Read the model definition and answer for the solid it produces. Units are mm, in the model's axes. A direction names the side the tool comes from. Coordinates: 2 decimals unless noted, no trailing zeros. Write each loop counter-clockwise with the first axis right and the second up, starting at its lowest first coordinate (ties: lowest second). Pieces come first, ordered by that corner, then holes. Notation, with made-up numbers: M -7,-13.5 L 32,-13.5 A28 cw 32,21.5 Z; hole C -2.5,11 d7. An arc over 180 degrees is marked long. Use a Markdown table: item, result. Add a question column.
from build123d import *

# Parameters (mm, degrees)
F1_DEPTH = 1.905
F3_DEPTH = 0.762
F4_R     = 4.445
F5_DEPTH = 3.048
F6_W     = 15.5236069113
F6_H     = 4.7940094955
F7_DEPTH = 0.762
F8_R     = 1.905
F9_DEPTH = 1.524


with BuildPart() as f1:
    # F0 (on Top) → F1 (new body)
    with BuildSketch(Plane.XY):
        with BuildLine():
            ThreePointArc((0, 10.16), (1.7642654851, 10.0056467706), (3.4749246562, 9.5472770272))
            Line((3.4749246562, 9.5472770272), (4.3436558202, 11.934096284))
            ThreePointArc((4.3436558202, 11.934096284), (2.2053318564, 12.5070584633), (0, 12.7))
            Line((0, 12.7), (0, 10.16))
        make_face()
        with BuildLine():
            ThreePointArc((-3.4749246562, 9.5472770272), (-1.7642654851, 10.0056467706), (0, 10.16))
            Line((0, 10.16), (0, 12.7))
            ThreePointArc((0, 12.7), (-2.2053318564, 12.5070584633), (-4.3436558202, 11.934096284))
            Line((-4.3436558202, 11.934096284), (-3.4749246562, 9.5472770272))
        make_face()
        with BuildLine():
            Line((4.3436558202, -11.934096284), (3.4749246562, -9.5472770272))
            ThreePointArc((3.4749246562, -9.5472770272), (0, -10.16), (-3.4749246562, -9.5472770272))
            Line((-3.4749246562, -9.5472770272), (-4.3436558202, -11.934096284))
            ThreePointArc((-4.3436558202, -11.934096284), (0, -12.7), (4.3436558202, -11.934096284))
        make_face()
        with BuildLine():
            Line((0, 0), (-1.5202795371, 4.1769336994))
            ThreePointArc((-1.5202795371, 4.1769336994), (-3.6411308369, 2.5495472596), (-4.445, 0))
            Line((-4.445, 0), (0, 0))
        make_face()
        with BuildLine():
            ThreePointArc((1.5202795371, -4.1769336994), (3.6411308369, -2.5495472596), (4.445, 0))
            ThreePointArc((4.445, 0), (3.6411308369, 2.5495472596), (1.5202795371, 4.1769336994))
            ThreePointArc((1.5202795371, 4.1769336994), (0.7718661497, 4.3774704621), (0, 4.445))
            Line((0, 4.445), (0, 0))
            Line((0, 0), (-4.445, 0))
            ThreePointArc((-4.445, 0), (-3.6411308369, -2.5495472596), (-1.5202795371, -4.1769336994))
            ThreePointArc((-1.5202795371, -4.1769336994), (0, -4.445), (1.5202795371, -4.1769336994))
        make_face()
        with BuildLine():
            Line((3.4749246562, -9.5472770272), (1.5202795371, -4.1769336994))
            ThreePointArc((1.5202795371, -4.1769336994), (0, -4.445), (-1.5202795371, -4.1769336994))
            Line((-1.5202795371, -4.1769336994), (-3.4749246562, -9.5472770272))
            ThreePointArc((-3.4749246562, -9.5472770272), (0, -10.16), (3.4749246562, -9.5472770272))
        make_face()
        with BuildLine():
            Line((0, 0), (0, 4.445))
            ThreePointArc((0, 4.445), (-0.7718661497, 4.3774704621), (-1.5202795371, 4.1769336994))
            Line((-1.5202795371, 4.1769336994), (0, 0))
        make_face()
        with BuildLine():
            ThreePointArc((-1.5202795371, 4.1769336994), (-0.7718661497, 4.3774704621), (0, 4.445))
            Line((0, 4.445), (0, 10.16))
            ThreePointArc((0, 10.16), (-1.7642654851, 10.0056467706), (-3.4749246562, 9.5472770272))
            Line((-3.4749246562, 9.5472770272), (-1.5202795371, 4.1769336994))
        make_face()
        with BuildLine():
            ThreePointArc((0, 4.445), (0.7718661497, 4.3774704621), (1.5202795371, 4.1769336994))
            Line((1.5202795371, 4.1769336994), (3.4749246562, 9.5472770272))
            ThreePointArc((3.4749246562, 9.5472770272), (1.7642654851, 10.0056467706), (0, 10.16))
            Line((0, 10.16), (0, 4.445))
        make_face()
    extrude(amount=F1_DEPTH)

    # F2 (on face) → F3 (join)
    with BuildSketch(Plane.XY.offset(1.905)):
        with BuildLine():
            Line((3.4749246562, 9.5472770272), (4.3436558202, 11.934096284))
            ThreePointArc((4.3436558202, 11.934096284), (0, 12.7), (-4.3436558202, 11.934096284))
            Line((-4.3436558202, 11.934096284), (-3.4749246562, 9.5472770272))
            ThreePointArc((-3.4749246562, 9.5472770272), (0, 10.16), (3.4749246562, 9.5472770272))
        make_face()
        with BuildLine():
            ThreePointArc((-4.3436558202, -11.934096284), (0, -12.7), (4.3436558202, -11.934096284))
            Line((4.3436558202, -11.934096284), (3.4749246562, -9.5472770272))
            ThreePointArc((3.4749246562, -9.5472770272), (0, -10.16), (-3.4749246562, -9.5472770272))
            Line((-3.4749246562, -9.5472770272), (-4.3436558202, -11.934096284))
        make_face()
    extrude(amount=F3_DEPTH)

    # F4 (on face) → F5 (join)
    with BuildSketch(Plane.XY.offset(1.905)):
        Circle(F4_R)
    extrude(amount=F5_DEPTH)

    # F6 (on face) → F7 (join)
    with BuildSketch(Plane.XY.offset(4.953)):
        Rectangle(F6_W, F6_H)
    extrude(amount=-F7_DEPTH)

    # F8 (on face) → F9 (join)
    with BuildSketch(Plane(origin=(0, 0, 0), x_dir=(1, 0, 0), z_dir=(0, 0, -1))):
        Circle(F8_R)
    extrude(amount=F9_DEPTH)


solid = f1.part
Item 1: For faces 1 (the flat face through (0, 0, -1.524)), 2 (the flat face through (0, -11, 2.667)), 3 (the flat face through (0, 11, 2.667)), determine the directions among +Z, -Z, +X, -X, +Y, -Y from which every point of the face is accessible in a straight line to the end or side of a thin tool.
Item 2: Find section C-C on y = -3.25. Give the vertices of the cut face in (x, z) (3 decimals).
Item 3: Determine the mould class of faces 4 (the cylindrical face through (-0.41, 1.86, -0.75)), 5 (the flat face through (0, -7, 1.905)), 6 (the flat face through (-6, 0, 4.191)) for opening direction Y: pulls with the +Y half, pulls with the -Y half, needs draft (parallel to the pull), parting line crosses it, or undercut.
Item 4: Find section A-A on z = 0.5. Give the vertices of the cut face in (x, y) (3 decimals).
Item 5: Consider probe 1 along Z at (x, y) = (-5.25, 1); probe 2 along Z at (x, y) = (0, -11); probe 3 along Y at (x, z) = (0, -1) (3 decimals). Determine where each line is inside the solid, lowest interval first.
Item 6: Find section D-D on x = -5.75. Give the vertices of the cut face in (y, z), then the cut area to 3 significant figures.
Item 7: Find section B-B on x = 3. Give the vertices of the cut face in (y, z) (3 decimals).
Item 8: Each of these flat-tipped pins is pushed along its axis until it touches: pin 1 (0.6 mm diameter, centred on x = 5.5, z = 4.5, fed in from +Y); pin 2 (1.5 mm diameter, centred on x = 3.5, z = 1, fed in from +Y); pin 3 (5 mm diameter, centred on x = 1, y = 8, fed in from +Z). Where does it stop, or does it pass through?
Geometry says:
| question | item | result |
|---|---|---|
| 1 | face 1 | -Z, +X, -X, +Y, -Y |
| 1 | face 2 | +Z, +X, -X, -Y |
| 1 | face 3 | +Z, +X, -X, +Y |
| 2 | outline | M -3.032,0 L 3.032,0 L 3.032,4.953 L -3.032,4.953 Z |
| 3 | face 4 | parting line crosses it |
| 3 | face 5 | undercut |
| 3 | face 6 | needs draft |
| 4 | outline | M -4.344,-11.934 A12.7 ccw 4.344,-11.934 L 1.52,-4.177 A4.445 ccw 1.52,4.177 L 4.344,11.934 A12.7 ccw -4.344,11.934 L -1.52,4.177 A4.445 ccw -1.52,-4.177 Z |
| 5 | probe 1 | z = 4.19 to 4.95 |
| 5 | probe 2 | z = 0 to 2.67 |
| 5 | probe 3 | y = -1.905 to 1.905 |
| 6 | outline | M -2.4,4.19 L 2.4,4.19 L 2.4,4.95 L -2.4,4.95 Z |
| 6 | area | 3.65 mm2 |
| 7 | outline | M -12.341,0 L -8.242,0 L -8.242,1.905 L -9.707,1.905 L -9.707,2.667 L -12.341,2.667 Z; M -3.28,0 L 3.28,0 L 3.28,4.953 L -3.28,4.953 Z; M 8.242,0 L 12.341,0 L 12.341,2.667 L 9.707,2.667 L 9.707,1.905 L 8.242,1.905 Z |
| 8 | pin 1 | stops at y = 2.4 |
| 8 | pin 2 | stops at y = 12.4 |
| 8 | pin 3 | stops at z = 2.67 |
